from build123d import *


with BuildPart() as part:
    # Sketch1 → Revolve1 (revolve)
    with BuildSketch(Plane.XY):
        with BuildLine():
            Line((0, 0), (0, 2))
            Line((0, 2), (-19.5, 2))
            ThreePointArc((-19.5, 2), (-23.389087297, 0.389087297), (-25, -3.5))
            Line((-25, -3.5), (-25, -9.3))
            Line((-25, -9.3), (-24, -9.3))
            Line((-24, -9.3), (-24, -4.3))
            Line((-24, -4.3), (-23, -4.3))
            Line((-23, -4.3), (-23, -3.5))
            ThreePointArc((-23, -3.5), (-21.974873734, -1.025126266), (-19.5, 0))
            Line((-19.5, 0), (0, 0))
        make_face()
    revolve(axis=Axis((0, 0, 0), (0, -1, 0)))


solid = part.part
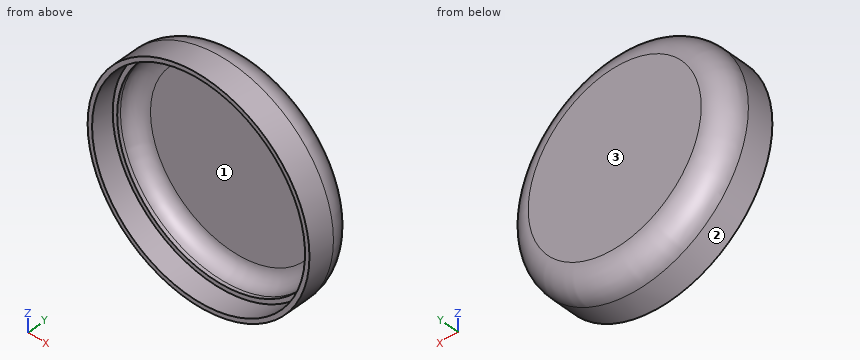
Could you check a few things on this model? Use its own coordinates, in mm. Face numbers are marked on the shaded views. Give positions to 0.01 mm unless a question says otherwise; leave off trailing zeros. Order: outer loops, then holes, each group sorted by start corner. A loop starts at its lowest first (then second) coordinate and runs counter-clockwise, first axis right, second up. Notation, with made-up numbers: (23.5, -18) -> (64.5, -18) arc R23 cw to (64.5, -1) -> close; hole circle Ø1 at (45, 88.5). An arc over 180 degrees is marked (long way). Answer in a Markdown table with one row per item. Add a question column.
Item 1: We'd pull the mould along X, two halves only. Please class the marked faces 1, 2 and 3: pulls with the +X half, pulls with the -X half, needs draft (parallel to the pull), parting line crosses it, or undercut.
Item 2: I'm going to push flat-ended pins straight in: P1, Ø2, axis at x = -4, y = 0.5, coming from the +Z side; P2, Ø5, axis at x = -1, z = 5, coming from the -Y side; P3, Ø4, axis at x = -11.5, y = -6, coming from the -Z side. Where does each tip first touch, or does it pass through?
Item 3: Imagine slicing it at D-D (y = -1.75). List the corners of the cut face in (x, z) for me.
Item 4: Imagine slicing it at A-A (z = 0). List the corners of the cut face in (x, y) for me, and give its area (3 significant figures).
Item 5: Imagine slicing it at C-C (y = -8.5). List the corners of the cut face in (x, z) for me, and give its area (3 significant figures).
Item 6: Imagine slicing it at B-B (x = 0). List the corners of the cut face in (y, z) for me, and give its area (3 significant figures).
Item 7: Please list where these lines run through material, in increasing order: probe 1 along X at (y, z) = (-5.75, 0); probe 2 along X at (y, z) = (-3.8, 0).
Result:
| question | item | result |
|---|---|---|
| 1 | face 1 | undercut |
| 1 | face 2 | parting line crosses it |
| 1 | face 3 | needs draft |
| 2 | P1 | z = 23.8 |
| 2 | P2 | y = 0 |
| 2 | P3 | z = -23.12 |
| 3 | outline | circle Ø49.43 at (0, 0); hole circle Ø45.06 at (0, 0) |
| 4 | outline | (-25, -9.3) -> (-24, -9.3) -> (-24, -4.3) -> (-23, -4.3) -> (-23, -3.5) arc R3.5 cw to (-19.5, 0) -> (19.5, 0) arc R3.5 cw to (23, -3.5) -> (23, -4.3) -> (24, -4.3) -> (24, -9.3) -> (25, -9.3) -> (25, -3.5) arc R5.5 ccw to (19.5, 2) -> (-19.5, 2) arc R5.5 ccw to (-25, -3.5) -> close |
| 4 | area | 119 mm2 |
| 5 | outline | circle Ø50 at (0, 0); hole circle Ø48 at (0, 0) |
| 5 | area | 154 mm2 |
| 6 | outline | (-9.3, -25) -> (-3.5, -25) arc R5.5 ccw to (2, -19.5) -> (2, 19.5) arc R5.5 ccw to (-3.5, 25) -> (-9.3, 25) -> (-9.3, 24) -> (-4.3, 24) -> (-4.3, 23) -> (-3.5, 23) arc R3.5 cw to (0, 19.5) -> (0, -19.5) arc R3.5 cw to (-3.5, -23) -> (-4.3, -23) -> (-4.3, -24) -> (-9.3, -24) -> close |
| 6 | area | 119 mm2 |
| 7 | probe 1 | -25 to -24, 24 to 25 |
| 7 | probe 2 | -25 to -23, 23 to 25 |
